```python
from build123d import *

# Parameters (mm, degrees)
F0_W = 25.4
F0_H = 25.4


with BuildPart() as f2:
    # F0 (on Top) → F2 section 0
    with BuildSketch(Plane.XY, mode=Mode.PRIVATE) as f2_s0:
        Rectangle(F0_W, F0_H)
    loft([f2_s0.sketch, Vertex(0, 0, 17.960512)])

    # F0 (on Top) → F3 section 0
    with BuildSketch(Plane.XY, mode=Mode.PRIVATE) as f3_s0:
        Rectangle(F0_W, F0_H)
    loft([f3_s0.sketch, Vertex(0, 0, -17.960512)])


solid = f2.part
```
Design review of the part built by this model. Coordinates are the model's own, in mm. Give positions to 0.01 mm unless a question says otherwise; leave off trailing zeros. Write each loop counter-clockwise with the first axis right and the second up, starting at its lowest first coordinate (ties: lowest second). Pieces come first, ordered by that corner, then holes.
(1) Clearance check with flat-ended pins moving along their axes: pin 1 Ø5 at (x, z) = (1.5, -7.5) entering from +Y; pin 2 Ø1.5 at (x, y) = (-6.5, -9) entering from -Z; pin 3 Ø8 at (y, z) = (-10, 7.5) entering from +X. State where each tip first meets the part, or that it passes through.
Checked values:
pin 1: stops at y = 9.16
pin 2: stops at z = -6.29
pin 3: stops at x = 10.23
(2) Add section D-D (z = -1). Give the boundary of the cut face in (x, y).
Checked values:
outline: (-11.99, -11.99) - (11.99, -11.99) - (11.99, 11.99) - (-11.99, 11.99) - close
(3) Add section A-A (x = 8.5). Give the boundary of the cut face in (y, z), and give its area (3 significant figures).
Checked values:
outline: (-12.7, 0) - (-8.5, -5.94) - (8.5, -5.94) - (12.7, 0) - (8.5, 5.94) - (-8.5, 5.94) - close
area: 252 mm2
(4) Add section B-B (y = -10.75). Give the boundary of the cut face in (x, z), and give its area (3 significant figures).
Checked values:
outline: (-12.7, 0) - (-10.75, -2.76) - (10.75, -2.76) - (12.7, 0) - (10.75, 2.76) - (-10.75, 2.76) - close
area: 129 mm2
(5) Wall thickness on line 1 along Z through (x, y) = (-5.5, -6); line 2 along Z through (x, y) = (10.75, -6.75); line 3 along X through (y, z) = (-5.5, -2): over which ranges is each line inside the solid? List them lowest first.
Checked values:
line 1: z = -9.48 to 9.48
line 2: z = -2.76 to 2.76
line 3: x = -11.29 to 11.29
(6) Add section C-C (z = -13). Give the boundary of the cut face in (x, y).
Checked values:
outline: (-3.51, -3.51) - (3.51, -3.51) - (3.51, 3.51) - (-3.51, 3.51) - close
